Geometry: see drawing. Coordinates: mm, zero at the bounding-box minimum. Coordinates: 2 decimals unless noted, no trailing zeros. Loops run counter-clockwise (first coordinate to the right, second up) from the corner with the lowest first, then second, coordinate; pieces in that order, holes last.
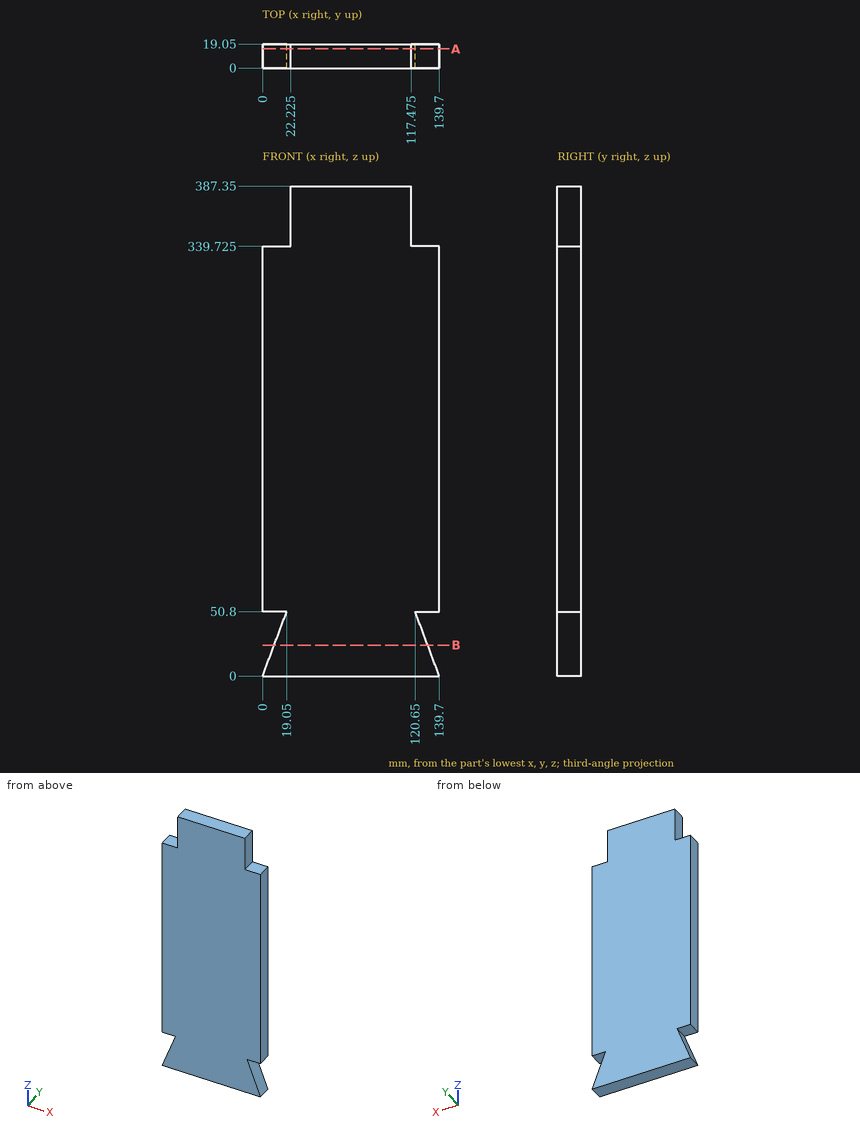
Item 1: Line query: L1, parallel to Z at x = 20, y = 18.25 (3 decimals); L2, parallel to X at y = 15, z = 358.5 (3 decimals); L3, parallel to X at y = 17.5, z = 48.5. Output: solid intervals per line, ascending.
Result:
L1: z = 0 to 339.725
L2: x = 22.225 to 117.475
L3: x = 18.19 to 121.51
Item 2: Section query B-B (z = 24.5). Output: boundary loops of the cut face in (x, y).
Result:
outline: (9.19, 0) - (130.51, 0) - (130.51, 19.05) - (9.19, 19.05) - close
Item 3: Contact query for flat-ended pins moving along their axis: P1, Ø5.5, axis at y = 12.5, z = 373, coming from the -X side (3 decimals); P2, Ø5.5, axis at x = 132.5, y = 5.5, coming from the +Z side (3 decimals). Output: stop coordinate, or through.
Result:
P1: stops at x = 22.225
P2: stops at z = 339.725
Item 4: Section query A-A (y = 15.25). Output: boundary loops of the cut face in (x, z) (3 decimals), then the cut area to 3 significant figures.
Result:
outline: (0, 0) - (139.7, 0) - (120.65, 50.8) - (139.7, 50.8) - (139.7, 339.725) - (117.475, 339.725) - (117.475, 387.35) - (22.225, 387.35) - (22.225, 339.725) - (0, 339.725) - (0, 50.8) - (19.05, 50.8) - close
area: 51,000 mm2
